Geometry: final body of the model. Coordinates: model frame, mm. A direction names the side the tool comes from. Give positions to 0.01 mm unless a question says otherwise; leave off trailing zeros. Write each loop counter-clockwise with the first axis right and the second up, starting at its lowest first coordinate (ties: lowest second). Pieces come first, ordered by that corner, then holes. Notation, with made-up numbers: (28, 29.5) -> (74, 29.5) arc R14 ccw to (74, 43.5) -> close; hole circle Ø2 at (76.25, -27). An arc over 180 degrees is marked (long way). Use CSV: the item, a comma, the result in double quotes. Start each with the question number.
1) Section C-C (z = -19). Output: boundary loops of the cut face in (x, y).
2) Section B-B (x = 0). Output: boundary loops of the cut face in (y, z), plus the area to 3 significant figures.
3) Section A-A (y = 17.5). Output: boundary loops of the cut face in (x, z), plus the area to 3 significant figures.
4) Set-up query: faces 1 (the face through (0, 16, 0)), 2 (the face through (0, 16, -24.6)). Return all of +Z, -Z, +X, -X, +Y, -Y with unobstructed straight access to the full face (end or side cutting, diameter ignored); none if empty.
5) Contact query for flat-ended pins moving along their axis: P1, Ø1.5, axis at y = 19, z = -20, coming from the -X side; P2, Ø1.5, axis at x = 2, z = -13.5, coming from the +Y side; P3, Ø1.5, axis at x = 1, z = -7, coming from the +Y side; P4, Ø1.5, axis at x = -1.5, z = -13, coming from the -Y side. Output: stop coordinate, or through.
6) Material intervals for line 1 (Z direction, x = -0.1, y = 15.8); line 2 (Z direction, x = -0.4, y = 15.1); line 3 (Y direction, x = 0, z = -11.75), sorted ascending. Write a range as [from, to].
```python
from build123d import *

# Parameters (mm, degrees)
SKETCH1_R           = 1
BASE_EXTRUDE_DEPTH  = 24.2
SKETCH2_R           = 2.81
BOSS_EXTRUDE1_DEPTH = 1
FILLET1_R           = 0.3
SKETCH3_R           = 2.05
BOSS_EXTRUDE2_DEPTH = 0.4
FILLET2_R           = 0.3


with BuildPart() as part:
    # Sketch1 → Base-Extrude (new body)
    with BuildSketch(Plane.XY):
        with Locations((0, 17.5)):
            Circle(SKETCH1_R)
    extrude(amount=-BASE_EXTRUDE_DEPTH)

    # Sketch2 → Boss-Extrude1 (add)
    with BuildSketch(Plane.XY):
        with Locations((0, 17.5)):
            Circle(SKETCH2_R)
    extrude(amount=BOSS_EXTRUDE1_DEPTH)

    # Fillet1
    fillet1_edges = [part.edges().sort_by_distance(p)[0] for p in [
        (-2.81, 17.5, 1),
    ]]
    fillet(fillet1_edges, radius=FILLET1_R)

    # Sketch3 → Boss-Extrude2 (add)
    with BuildSketch(Plane(origin=(0, 0, -24.2), x_dir=(-1, 0, 0), z_dir=(0, 0, -1))):
        with Locations((0, 17.5)):
            Circle(SKETCH3_R)
    extrude(amount=BOSS_EXTRUDE2_DEPTH)

    # Sketch4 → Cut-Revolve1 (revolve, cut)
    with BuildSketch(Plane(origin=(0, 0, -24.6), x_dir=(-1, 0, 0), z_dir=(0, 0, -1))):
        with BuildLine():
            Line((0.918394915, 17.104335014), (-0.918394915, 17.895664986))
            ThreePointArc((-0.918394915, 17.895664986), (-0.395664986, 16.581605085), (0.918394915, 17.104335014))
        make_face()
    revolve(axis=Axis((0.918394915, 17.895664986, -24.6), (-0.918394915, -0.395664986, 0)), mode=Mode.SUBTRACT)

    # Fillet2
    fillet2_edges = [part.edges().sort_by_distance(p)[0] for p in [
        (2.05, 17.5, -24.6),
    ]]
    fillet(fillet2_edges, radius=FILLET2_R)


solid = part.part
```
Answers follow:
1,outline,"circle Ø2 at (0, 17.5)"
2,outline,"(14.69, 0) -> (16.5, 0) -> (16.5, -24.2) -> (15.45, -24.2) -> (15.45, -24.3) arc R0.3 ccw to (15.75, -24.6) -> (16.5, -24.6) arc R1 cw to (18.5, -24.6) -> (19.25, -24.6) arc R0.3 ccw to (19.55, -24.3) -> (19.55, -24.2) -> (18.5, -24.2) -> (18.5, 0) -> (20.31, 0) -> (20.31, 0.7) arc R0.3 ccw to (20.01, 1) -> (14.99, 1) arc R0.3 ccw to (14.69, 0.7) -> close"
2,area,"54.0 mm^2"
3,outline,"(-2.81, 0) -> (-1, 0) -> (-1, -24.2) -> (-2.05, -24.2) -> (-2.05, -24.3) arc R0.3 ccw to (-1.75, -24.6) -> (-1, -24.6) arc R1 cw to (1, -24.6) -> (1.75, -24.6) arc R0.3 ccw to (2.05, -24.3) -> (2.05, -24.2) -> (1, -24.2) -> (1, 0) -> (2.81, 0) -> (2.81, 0.7) arc R0.3 ccw to (2.51, 1) -> (-2.51, 1) arc R0.3 ccw to (-2.81, 0.7) -> close"
3,area,"54.0 mm^2"
4,face 1,"none"
4,face 2,"-Z, +X, -X, +Y, -Y"
5,P1,"stops at x = -0.66"
5,P2,"passes through"
5,P3,"stops at y = 18.47"
5,P4,"stops at y = 16.84"
6,line 1,"z = [-24.6, -24.2], [0, 1]"
6,line 2,"z = [0, 1]"
6,line 3,"y = [16.5, 18.5]"
